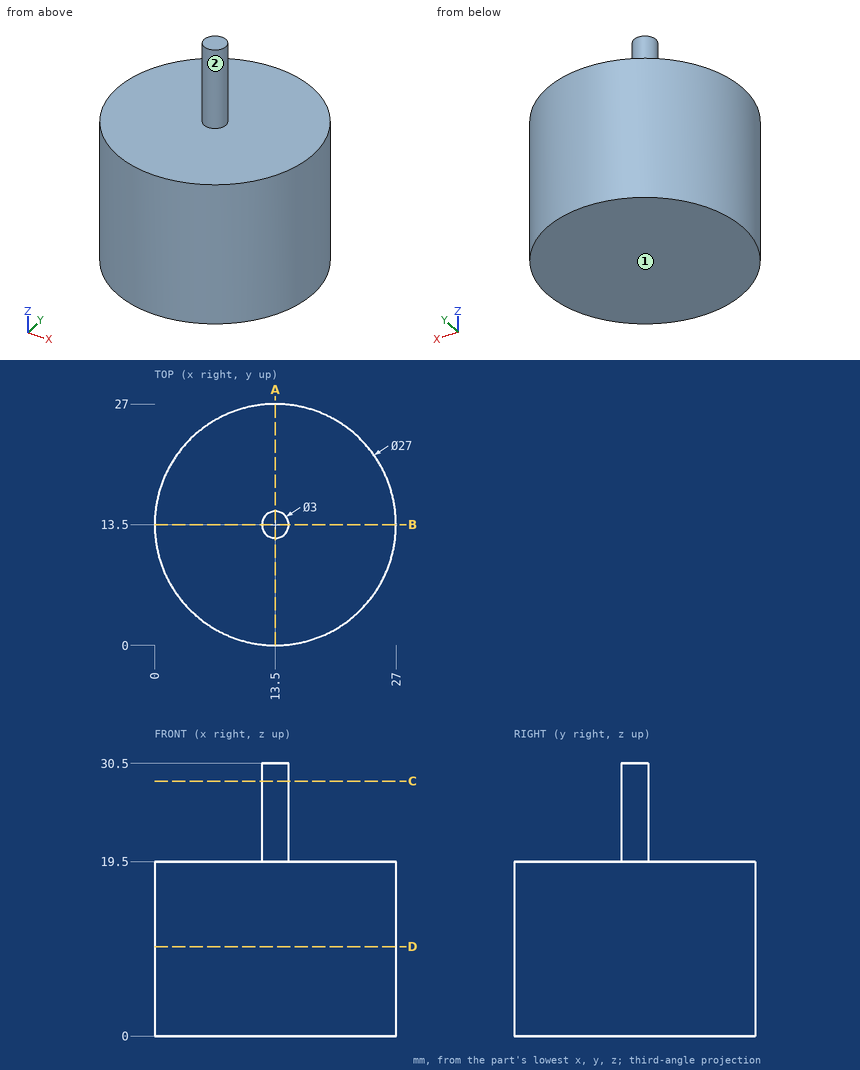
Verification items for this drawing (mm, ordinates from the low corner). A direction names the side the tool comes from. Give positions to 0.01 mm unless a question says otherwise; leave off trailing zeros. Loops run counter-clockwise (first coordinate to the right, second up) from the corner with the lowest first, then second, coordinate; pieces in that order, holes last. Notation, with made-up numbers: (58.5, 82.5) - (79.5, 82.5) arc R12 ccw to (79.5, 90.5) - close; hole circle Ø1 at (-11.5, -7). An arc over 180 degrees is marked (long way). Write item = value, one per line. Start each with the question number.
Q1. Tool access check on the marked faces 1 and 2. Record the directions out of +Z, -Z, +X, -X, +Y, -Y that give a thin tool (end or side, any length) a straight path to the whole face; none if there is none.
Q2. Cross-section at D-D, the plane z = 10. Enter the section's corners in (x, y), and give its area (3 significant figures).
Q3. Cross-section at A-A, the plane x = 13.5. Enter the section's corners in (y, z).
Q4. Thickness scan on line 1 (Z direction, x = 9.75, y = 13); line 2 (Y direction, x = 5.75, z = 12); line 3 (X direction, y = 25.25, z = 5.5). Record the ranges inside material, lowest first.
Q5. Depth check by flat-ended pin: P1, Ø3, axis at x = 10.5, z = 4, coming from the -Y side; P2, Ø1, axis at y = 23, z = 4, coming from the +X side; P3, Ø2, axis at x = 8, z = 14.5, coming from the -Y side; P4, Ø5, axis at x = 18, z = 26.5, coming from the +Y side. Enter the tip coordinate at first touch or a pass-through.
Q6. Cross-section at C-C, the plane z = 28.5. Enter the section's corners in (x, y), and give its area (3 significant figures).
Answer key:
q1.face_1 = -Z, +X, -X, +Y, -Y
q1.face_2 = +Z
q2.outline = circle Ø27 at (13.5, 13.5)
q2.area = 573 mm^2
q3.outline = (0, 0) - (27, 0) - (27, 19.5) - (15, 19.5) - (15, 30.5) - (12, 30.5) - (12, 19.5) - (0, 19.5) - close
q4.line_1 = 0 to 19.5
q4.line_2 = 2.45 to 24.55
q4.line_3 = 6.85 to 20.15
q5.P1 = 0.08
q5.P2 = 23.56
q5.P3 = 0.77
q5.P4 = through
q6.outline = circle Ø3 at (13.5, 13.5)
q6.area = 7.07 mm^2
